Geometry check sheet. Reference: the model listing, model coordinates, mm. Give positions to 0.01 mm unless a question says otherwise; leave off trailing zeros. Write each loop counter-clockwise with the first axis right and the second up, starting at its lowest first coordinate (ties: lowest second). Pieces come first, ordered by that corner, then holes.
(1) Cross-section at B-B (z = 3.7). Count the separate pieces of the cut face and the enclosed holes in it, and give its area (3 significant figures).
(2) Thickness scan on line 1 along X through (y, z) = (-1, 1.15); line 2 along Y through (x, z) = (24.5, 2.95); line 3 along Y through (x, z) = (26, 1.25). Record the ranges inside material, lowest first.
(3) Cross-section at A-A (y = -117). Record the boundary of the cut face in (x, z).
(4) Depth check by flat-ended pin: P1, Ø1, axis at y = -83.5, z = 2, coming from the -X side; P2, Ø8.5, axis at x = -12.7, y = 132.74, coming from the +Z side; P3, Ø1.5, axis at x = 5.5, z = 2.5, coming from the -Y side. Enter the tip coordinate at first touch or a pass-through.
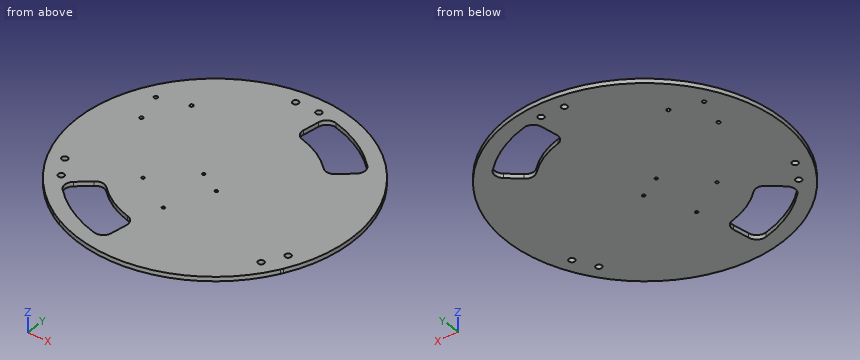
```python
from build123d import *

# Parameters (mm, degrees)
BOSS_EXTRUDE1_DEPTH          = 4.762
SKETCH5_R                    = 1.926649595
MOTOR_MOUNTING_HOLES_DEPTH   = 5.762
SKETCH7_R                    = 1.5875
ARDUINO_MOUNTING_HOLES_DEPTH = 5.762
SKETCH9_R                    = 3.2639
F_1_4_20_FEET_HOLES_DEPTH    = 5.762
HANDLES_DEPTH                = 5.762


with BuildPart() as part:
    # Sketch1 → Boss-Extrude1 (new body)
    with BuildSketch(Plane.XY):
        with BuildLine():
            ThreePointArc((-80.354757502, -125.742648182), (-74.6125, -129.23264088), (-68.718948913, -132.460585403))
            ThreePointArc((-68.718948913, -132.460585403), (41.077351206, -143.459931141), (128.412526716, -76.015285354))
            ThreePointArc((128.412526716, -76.015285354), (129.23264088, -74.6125), (130.03743155, -73.200867623))
            ThreePointArc((130.03743155, -73.200867623), (-36.155935906, 144.778620396), (-80.354757502, -125.742648182))
        make_face()
    extrude(amount=BOSS_EXTRUDE1_DEPTH)

    # Sketch5 → motor_mounting_holes (cut, through all)
    with BuildSketch(Plane.XY.offset(4.762)):
        with Locations((-81.719743632, 74.457252102)):
            Circle(SKETCH5_R)
        with Locations((-113.98799572, 65.811000014)):
            Circle(SKETCH5_R)
        with Locations((-105.341743632, 33.542747925)):
            Circle(SKETCH5_R)
    extrude(amount=-MOTOR_MOUNTING_HOLES_DEPTH, mode=Mode.SUBTRACT)

    # Sketch7 → arduino mounting holes (cut, through all)
    with BuildSketch(Plane(origin=(0, 0, 0), x_dir=(-1, 0, 0), z_dir=(0, 0, -1))):
        with Locations((-13.114276913, -15.277418882)):
            Circle(SKETCH7_R)
        with Locations((8.521314036, -62.911361657)):
            Circle(SKETCH7_R)
        with Locations((11.082472869, -1.307418882)):
            Circle(SKETCH7_R)
        with Locations((49.680700023, -37.681509395)):
            Circle(SKETCH7_R)
    extrude(amount=-ARDUINO_MOUNTING_HOLES_DEPTH, mode=Mode.SUBTRACT)

    # Sketch9 → 1/4-20 feet holes (cut, through all)
    with BuildSketch(Plane.XY.offset(4.762)):
        with Locations((121.309555388, -55.373407621)):
            Circle(SKETCH9_R)
        with Locations((108.609555388, -77.370452877)):
            Circle(SKETCH9_R)
        with Locations((-108.609555388, -77.370452877)):
            Circle(SKETCH9_R)
        with Locations((-121.309555388, -55.373407621)):
            Circle(SKETCH9_R)
        with Locations((-12.7, 132.743860498)):
            Circle(SKETCH9_R)
        with Locations((12.7, 132.743860498)):
            Circle(SKETCH9_R)
    extrude(amount=-F_1_4_20_FEET_HOLES_DEPTH, mode=Mode.SUBTRACT)

    # Sketch8 → handles (cut, through all)
    with BuildSketch(Plane.XY.offset(4.762)):
        with BuildLine():
            Line((21.318841652, 120.905159074), (18.219031169, 103.325260238))
            ThreePointArc((18.219031169, 103.325260238), (19.630613539, 96.141801354), (25.504227054, 91.771983211))
            ThreePointArc((25.504227054, 91.771983211), (47.625, 82.48891971), (66.724755289, 67.973300138))
            ThreePointArc((66.724755289, 67.973300138), (73.445935569, 65.071510694), (80.372784634, 67.440773943))
            Line((80.372784634, 67.440773943), (94.047518381, 78.915237986))
            ThreePointArc((94.047518381, 78.915237986), (97.666057076, 86.231232388), (94.734676371, 93.848620624))
            ThreePointArc((94.734676371, 93.848620624), (66.675, 115.484487595), (33.907951385, 128.966946668))
            ThreePointArc((33.907951385, 128.966946668), (25.845409309, 127.696902709), (21.318841652, 120.905159074))
        make_face()
        with BuildLine():
            Line((-94.047518381, -78.915237986), (-80.372784634, -67.440773943))
            ThreePointArc((-80.372784634, -67.440773943), (-73.445935569, -65.071510694), (-66.724755289, -67.973300138))
            ThreePointArc((-66.724755289, -67.973300138), (-47.625, -82.48891971), (-25.504227054, -91.771983211))
            ThreePointArc((-25.504227054, -91.771983211), (-19.630613539, -96.141801354), (-18.219031169, -103.325260238))
            Line((-18.219031169, -103.325260238), (-21.318841652, -120.905159074))
            ThreePointArc((-21.318841652, -120.905159074), (-25.845409309, -127.696902709), (-33.907951385, -128.966946668))
            ThreePointArc((-33.907951385, -128.966946668), (-66.675, -115.484487595), (-94.734676371, -93.848620624))
            ThreePointArc((-94.734676371, -93.848620624), (-97.666057076, -86.231232388), (-94.047518381, -78.915237986))
        make_face()
    extrude(amount=-HANDLES_DEPTH, mode=Mode.SUBTRACT)


solid = part.part
```
Reply:
1. separate pieces: 1
1. enclosed holes: 15
1. area: 63,800 mm2
2. line 1: x = -149.22 to -12.64, -9.53 to 149.22
2. line 2: y = -147.2 to 92.11, 126.67 to 147.2
2. line 3: y = -146.94 to 91.63, 127.79 to 146.94
3. outline: (-92.62, 0) - (-63.98, 0) - (-63.98, 4.76) - (-92.62, 4.76) - close; (-20.63, 0) - (92.62, 0) - (92.62, 4.76) - (-20.63, 4.76) - close
4. P1: stops at x = -124.01
4. P2: stops at z = 4.76
4. P3: stops at y = -149.15
